The listing builds one solid part. Answer for the finished solid, in the listing's coordinates (mm). Round coordinates to 2 decimals unless told otherwise and drop trailing zeros. Loops run counter-clockwise (first coordinate to the right, second up) from the corner with the lowest first, then second, coordinate; pieces in that order, holes last. Notation, with made-up numbers: (-9, 62) -> (24, 62) arc R23 cw to (24, 80) -> close; hole circle Ø2 at (-13.75, 22.25). An arc over 180 degrees is marked (long way). One line per question, with ' | ' between items.
from build123d import *

# Parameters (mm, degrees)
SKETCH1_R           = 1.5
BOSS_EXTRUDE1_DEPTH = 2.16
CHAMFER1_SIZE       = 0.25


with BuildPart() as part:
    # Sketch1 → Boss-Extrude1 (new body)
    with BuildSketch(Plane.XY):
        Polygon((2.72, 1.570392732), (0, 3.140785464), (-2.72, 1.570392732), (-2.72, -1.570392732), (0, -3.140785464), (2.72, -1.570392732), align=None)
        Circle(SKETCH1_R, mode=Mode.SUBTRACT)
    extrude(amount=BOSS_EXTRUDE1_DEPTH)

    # Chamfer1
    chamfer1_edges = [part.edges().sort_by_distance(p)[0] for p in [
        (-1.5, 0, 0),
        (-1.5, 0, 2.16),
    ]]
    chamfer(chamfer1_edges, length=CHAMFER1_SIZE)

    # Sketch2 → Cut-Revolve1 (revolve, cut)
    with BuildSketch(Plane(origin=(0, 0, 0), x_dir=(1, 0, 0), z_dir=(0, 1, 0))):
        with BuildLine():
            Line((-3.580128719, -0.636846199), (-4.500819954, -0.636846199))
            Line((-4.500819954, -0.636846199), (-4.500819954, 0.361239255))
            Line((-4.500819954, 0.361239255), (-2.72, 0.361239255))
            Line((-2.72, 0.361239255), (-2.72, 0))
            ThreePointArc((-2.72, 0), (-3.255115524, -0.176540297), (-3.580128719, -0.636846199))
        make_face()
        with BuildLine():
            Line((-2.72, -2.521239255), (-2.72, -2.16))
            ThreePointArc((-2.72, -2.16), (-3.255115524, -1.983459703), (-3.580128719, -1.523153801))
            Line((-3.580128719, -1.523153801), (-4.500819954, -1.523153801))
            Line((-4.500819954, -1.523153801), (-4.500819954, -2.521239255))
            Line((-4.500819954, -2.521239255), (-2.72, -2.521239255))
        make_face()
    revolve(axis=Axis((0, 0, 1.08), (0, 0, -1)), mode=Mode.SUBTRACT)


solid = part.part
Q1. Find the intervals of material crossed by line 1 (Y direction, x = 0.9, z = 0.95); line 2 (Y direction, x = 0.4, z = 0.4); line 3 (X direction, y = -0.5, z = 2.05), in increasing order. Write a range as from..to.
Numbers:
line 1: -2.62..-1.2, 1.2..2.62 | line 2: -2.91..-1.45, 1.45..2.91 | line 3: -2.72..-1.56, 1.56..2.72
Q2. For a pull along X with two mould halves and no side action, classify faces 1 (the face through (-1.341, 2.367, 1.065)), 2 (the face through (0, -2, 2.16)), 3 (the face through (-1.5, 0.07, 1.07)) as pulls with the +X half, pulls with the -X half, needs draft (parallel to the pull), parting line crosses it, or undercut.
Numbers:
face 1: pulls with the -X half | face 2: needs draft | face 3: undercut
Q3. Given pin 1 Ø2.5 at (x, y) = (0, 0) entering from +Z; pin 2 Ø1 at (y, z) = (2, 1.5) entering from -X, each flat-ended and moving along its own axis, determine where each tip first touches the part or whether it passes through.
Numbers:
pin 1: through | pin 2: x = -2.72
Q4. A cutting plane is placed at A-A on z = 1.65. Give the vertices of the cut face in (x, y).
Numbers:
outline: (-2.72, -1.57) -> (0, -3.14) -> (2.72, -1.57) -> (2.72, 1.57) -> (0, 3.14) -> (-2.72, 1.57) -> close; hole circle Ø3 at (0, 0)
